Input: part model. Units: mm. Frame: model coordinates. A direction names the side the tool comes from. Round coordinates to 2 decimals unless told otherwise and drop trailing zeros. Loops run counter-clockwise (first coordinate to the right, second up) from the corner with the lowest first, then second, coordinate; pieces in that order, holes last. Notation, with made-up numbers: (-25, -37) -> (-18, -37) arc R14 ccw to (-18, -25) -> close; hole circle Ø8 at (52, -38.75). An arc over 180 degrees is marked (long way). One line per question, with ' | ' between items. Start each with the question number.
Q1. Material intervals for L1, parallel to X at y = -5.5, z = 45.5; L2, parallel to X at y = -4, z = 27.5, sorted ascending.
Q2. Cut plane A-A on y = -4.5. Return loops of the section in (x, z).
Q3. Access query for faces 4 (the face through (61.25, -12, 37)), 5 (the face through (-55, -6.573, 37)), 6 (the face through (59, -6.573, 37)). Directions: +Z, -Z, +X, -X, +Y, -Y. A direction counts if a zero-diameter tool reaches every point of the face in a straight line with its end or side. Return the directions, or none.
Q4. Mould query, pull axis Y, two halves, no side actions, for faces 1 (the face through (1, 17, 37)), 2 (the face through (-56.75, 7, 37)), 3 (the face through (54.677, -4.454, 36.975)). Classes: pulls with the +Y half, pulls with the -Y half, needs draft (parallel to the pull), parting line crosses it, or undercut.
from build123d import *

# Parameters (mm, degrees)
ESTRUSIONE_ESTRUSIONE1_DEPTH = 75


with BuildPart() as part:
    # Schizzo1 → Estrusione-Estrusione1 (new body)
    with BuildSketch(Plane.XY):
        with BuildLine():
            Line((-56.75, 17), (61.25, 17))
            Line((61.25, 17), (61.25, -2.426773282))
            Line((61.25, -2.426773282), (56.75, -2.426773282))
            ThreePointArc((56.75, -2.426773282), (54.676773282, -4.5), (56.75, -6.573226718))
            Line((56.75, -6.573226718), (61.25, -6.573226718))
            Line((61.25, -6.573226718), (61.25, -17))
            Line((61.25, -17), (-56.75, -17))
            Line((-56.75, -17), (-56.75, -6.573226718))
            Line((-56.75, -6.573226718), (-52.25, -6.573226718))
            ThreePointArc((-52.25, -6.573226718), (-50.176773282, -4.5), (-52.25, -2.426773282))
            Line((-52.25, -2.426773282), (-56.75, -2.426773282))
            Line((-56.75, -2.426773282), (-56.75, 17))
        make_face()
    extrude(amount=ESTRUSIONE_ESTRUSIONE1_DEPTH)


solid = part.part
Results:
1) L1: -50.43 to 54.93 | L2: -50.24 to 54.74
2) outline: (-50.18, 0) -> (54.68, 0) -> (54.68, 75) -> (-50.18, 75) -> close
3) face 4: +Z, -Z, +X, +Y, -Y | face 5: +Z, -Z, -X | face 6: +Z, -Z, +X
4) face 1: pulls with the +Y half | face 2: needs draft | face 3: undercut
